Source: CAD feature listing. Evaluate the final solid. Frame: model axes, mm. A direction names the side the tool comes from. Round coordinates to 2 decimals unless told otherwise and drop trailing zeros. Loops run counter-clockwise (first coordinate to the right, second up) from the corner with the lowest first, then second, coordinate; pieces in that order, holes last. Notation, with made-up numbers: M -24.75,-28 L 1.25,-28 A13 ccw 1.25,-5 Z; hole C 41.25,28.5 d6. An arc over 180 degrees is marked long. Write each question's results on one line, items separated by ' | '. Start each with the question number.
1. Section A-A on y = 11. Output: boundary loops of the cut face in (x, z).
2. Section B-B on z = -12. Output: boundary loops of the cut face in (x, y), and give its area (3 significant figures).
3. Contact query for flat-ended pins moving along their axis: pin 1 Ø11 at (x, y) = (15, 11) entering from +Z; pin 2 Ø8 at (x, z) = (10.5, -22.5) entering from +Y. Output: stop coordinate, or through.
4. Section C-C on x = 15. Output: boundary loops of the cut face in (y, z), and give its area (3 significant figures).
5. Ray query, line 1 (X direction, y = 0.75, z = -12); line 2 (Z direction, x = 26.5, y = 16); line 3 (X direction, y = 11, z = 1.25). Return the intervals inside material, ascending.
6. Section D-D on y = 30.5. Output: boundary loops of the cut face in (x, z), and give its area (3 significant figures).
7. Set-up query: faces 5 (the flat face through (15, 18, -27)), 6 (the flat face through (15, 20, 3)). Return all of +Z, -Z, +X, -X, +Y, -Y with unobstructed straight access to the full face (end or side cutting, diameter ignored); none if empty.
8. Draft query along Z for faces 1 (the flat face through (15, 33, 1)), 2 (the flat face through (15, 3, -14)), 3 (the flat face through (15, 20, -30)), 4 (the flat face through (15, 18, 0)). Return one class per face: released by +Z, released by -Z, zero draft, split by the parting line, or undercut.
from build123d import *

# Parameters (mm, degrees)
SKETCH1_W           = 30
SKETCH1_H           = 30
SKETCH1_R           = 1.15
BOSS_EXTRUDE1_DEPTH = 3
SKETCH2_W           = 30
SKETCH2_H           = 3
BOSS_EXTRUDE2_DEPTH = 30
CUT_EXTRUDE1_REACH  = 55.749
SKETCH3_R           = 6
SKETCH4_W           = 30
SKETCH4_H           = 33
SKETCH4_R           = 6
BOSS_EXTRUDE3_DEPTH = 3


with BuildPart() as part:
    # Sketch1 → Boss-Extrude1 (new body)
    with BuildSketch(Plane(origin=(0, 0, 0), x_dir=(1, 0, 0), z_dir=(0, 1, 0))):
        with Locations((15, 15)):
            Rectangle(SKETCH1_W, SKETCH1_H)
        with Locations(Location((5.999988, 12, 0), (0, 0, 270))):
            Circle(SKETCH1_R, mode=Mode.SUBTRACT)
        with Locations(Location((23.999988, 12, 0), (0, 0, 270))):
            Circle(SKETCH1_R, mode=Mode.SUBTRACT)
    extrude(amount=BOSS_EXTRUDE1_DEPTH)

    # Sketch2 → Boss-Extrude2 (add)
    with BuildSketch(Plane(origin=(0, 3, 0), x_dir=(1, 0, 0), z_dir=(0, 1, 0))):
        with Locations((15, 28.5)):
            Rectangle(SKETCH2_W, SKETCH2_H)
    extrude(amount=BOSS_EXTRUDE2_DEPTH)

    # Sketch3 → Cut-Extrude1 (cut, up to next)
    with BuildSketch(Plane(origin=(0, 0, -30), x_dir=(-1, 0, 0), z_dir=(0, 0, -1)), mode=Mode.PRIVATE) as cut_extrude1_sk1:
        with Locations((-15, 11)):
            Circle(SKETCH3_R)
    cut_extrude1_tool1 = extrude(cut_extrude1_sk1.sketch, amount=-CUT_EXTRUDE1_REACH, mode=Mode.PRIVATE) & part.part
    add(cut_extrude1_tool1.solids().sort_by_distance((15, 11, -30))[0], mode=Mode.SUBTRACT)

    # Sketch4 → Boss-Extrude3 (add)
    with BuildSketch(Plane.XY):
        with Locations((15, 16.5)):
            Rectangle(SKETCH4_W, SKETCH4_H)
        with Locations(Location((15, 11, 0), (0, 0, 180))):
            Circle(SKETCH4_R, mode=Mode.SUBTRACT)
    extrude(amount=BOSS_EXTRUDE3_DEPTH)


solid = part.part
Taken from the geometry:
1) outline: M 0,-30 L 9,-30 L 9,-27 L 0,-27 Z; M 0,0 L 9,0 L 9,3 L 0,3 Z; M 21,-30 L 30,-30 L 30,-27 L 21,-27 Z; M 21,0 L 30,0 L 30,3 L 21,3 Z
2) outline: M 0,0 L 4.85,0 L 4.85,3 L 0,3 Z; M 7.15,0 L 22.85,0 L 22.85,3 L 7.15,3 Z; M 25.15,0 L 30,0 L 30,3 L 25.15,3 Z | area: 76.2 mm^2
3) pin 1: through | pin 2: y = 3
4) outline: M 0,-30 L 5,-30 L 5,-27 L 3,-27 L 3,0 L 5,0 L 5,3 L 0,3 Z; M 17,-30 L 33,-30 L 33,-27 L 17,-27 Z; M 17,0 L 33,0 L 33,3 L 17,3 Z | area: 207 mm^2
5) line 1: 0 to 4.85, 7.15 to 22.85, 25.15 to 30 | line 2: -30 to -27, 0 to 3 | line 3: 0 to 9, 21 to 30
6) outline: M 0,-30 L 30,-30 L 30,-27 L 0,-27 Z; M 0,0 L 30,0 L 30,3 L 0,3 Z | area: 180 mm^2
7) face 5: +X, -X, +Y | face 6: +Z, +X, -X, +Y, -Y
8) face 1: zero draft | face 2: undercut | face 3: released by -Z | face 4: undercut
